```python
from build123d import *

# Parameters (mm, degrees)
F1_DEPTH  = 37
F2_R      = 2
F3_DEPTH  = 25.4
F4_R      = 5
F2_W      = 38.9878123262
F2_H      = 37
F5_DEPTH  = 10
F6_R      = 3
F7_DEPTH  = 10
F9_DEPTH  = 25.4
F11_DEPTH = 25.4


with BuildPart() as f1:
    # F0 (on Front) → F1 (new body)
    with BuildSketch(Plane.XZ):
        with BuildLine():
            Line((-75.544338002, 59.8869249225), (-114.5321503282, 59.8869249225))
            Line((-114.5321503282, 59.8869249225), (-114.5509034395, 46.8869249225))
            Line((-114.5509034395, 46.8869249225), (-110.5809034395, 46.8811980108))
            ThreePointArc((-110.5809034395, 46.8811980108), (-95.048956228, 54.9422402402), (-79.514338002, 46.8863465853))
            Line((-79.514338002, 46.8863465853), (-75.544338002, 46.8863465853))
            Line((-75.544338002, 46.8863465853), (-75.544338002, 59.8869249225))
        make_face()
    extrude(amount=F1_DEPTH)

    # F2 (on face) → F3 (cut)
    with BuildSketch(Plane.XY.offset(59.8869249225)):
        with Locations((-95.0382441651, -18.5)):
            Circle(F2_R)
    extrude(amount=-F3_DEPTH, mode=Mode.SUBTRACT)

    # F4 (on face) + F2 (on face) → F5 (join)
    with BuildSketch(Plane.XY.offset(59.8869249225)):
        with BuildLine():
            Line((-75.544338002, -37), (-61.284338002, -37))
            ThreePointArc((-61.284338002, -37), (-56.4913599263, -18.5), (-61.284338002, 0))
            Line((-61.284338002, 0), (-75.544338002, 0))
            Line((-75.544338002, 0), (-75.544338002, -37))
        make_face()
        with Locations((-69.575338002, -18.5)):
            Circle(F4_R, mode=Mode.SUBTRACT)
        with BuildLine():
            Line((-128.7921503282, -37), (-114.5321503282, -37))
            Line((-114.5321503282, -37), (-114.5321503282, 0))
            Line((-114.5321503282, 0), (-128.7921503282, 0))
            ThreePointArc((-128.7921503282, 0), (-133.6226710865, -18.5), (-128.7921503282, -37))
        make_face()
        with Locations((-120.4896494746, -18.5)):
            Circle(F4_R, mode=Mode.SUBTRACT)
    with BuildSketch(Plane.XY.offset(59.8869249225)):
        with Locations((-95.0382441651, -18.5)):
            Rectangle(F2_W, F2_H)
        with Locations((-95.0382441651, -18.5)):
            Circle(F2_R, mode=Mode.SUBTRACT)
    extrude(amount=F5_DEPTH)

    # F6 (on face) → F7 (join)
    with BuildSketch(Plane.XY.offset(69.8869249225)):
        with BuildLine():
            Line((-75.544338002, 0), (-114.5321503282, 0))
            Line((-114.5321503282, 0), (-114.5321503282, -8.38))
            ThreePointArc((-114.5321503282, -8.38), (-108.9808401176, -18.5), (-114.5321503282, -28.62))
            Line((-114.5321503282, -28.62), (-114.5321503282, -37))
            Line((-114.5321503282, -37), (-75.544338002, -37))
            Line((-75.544338002, -37), (-75.544338002, -28.62))
            ThreePointArc((-75.544338002, -28.62), (-81.0956482126, -18.5), (-75.544338002, -8.38))
            Line((-75.544338002, -8.38), (-75.544338002, 0))
        make_face()
        with Locations((-95.0382441651, -18.5)):
            Circle(F6_R, mode=Mode.SUBTRACT)
    extrude(amount=F7_DEPTH)

    # F8 (on face) → F9 (cut)
    with BuildSketch(Plane(origin=(0, 0, 0), x_dir=(-1, 0, 0), z_dir=(0, 1, 0))):
        with BuildLine():
            ThreePointArc((75.544338002, 69.8869249225), (95.0382441651, 75.2681017907), (114.5321503282, 69.8869249225))
            Line((114.5321503282, 69.8869249225), (114.5321503282, 79.8869249225))
            Line((114.5321503282, 79.8869249225), (75.544338002, 79.8869249225))
            Line((75.544338002, 79.8869249225), (75.544338002, 69.8869249225))
        make_face()
    extrude(amount=-F9_DEPTH, mode=Mode.SUBTRACT)

    # F10 (on face) → F11 (cut)
    with BuildSketch(Plane.XZ.offset(37)):
        with BuildLine():
            ThreePointArc((-114.5321503282, 69.8869249225), (-95.0382441651, 75.2681017907), (-75.544338002, 69.8869249225))
            Line((-75.544338002, 69.8869249225), (-75.544338002, 79.8869249225))
            Line((-75.544338002, 79.8869249225), (-114.5321503282, 79.8869249225))
            Line((-114.5321503282, 79.8869249225), (-114.5321503282, 69.8869249225))
        make_face()
    extrude(amount=-F11_DEPTH, mode=Mode.SUBTRACT)


solid = f1.part
```
Check sheet for the modelled part. Datum: model origin and axes. Units: mm. A direction names the side the tool comes from. Round coordinates to 2 decimals unless told otherwise and drop trailing zeros. Loops run counter-clockwise (first coordinate to the right, second up) from the corner with the lowest first, then second, coordinate; pieces in that order, holes last. Notation, with made-up numbers: (68.25, -6.5) -> (77.25, -6.5) arc R23 cw to (77.25, 7.5) -> close; hole circle Ø8 at (41.5, -18). An arc over 180 degrees is marked (long way). Write item = value, one per line. Start each with the question number.
1) Sectioned sample at C-C, the plane z = 49. Record the cut outline in (x, y), plus the area to 3 significant figures.
2) Sectioned sample at B-B, the plane y = -18.5. State how many separate pieces and enclosed holes the cut face has, plus the area to 3 significant figures.
3) Release check for a two-part mould opening along X. For faces 1 (the flat face through (-75.544, -18, 53)), 2 (the cylindrical face through (-97.419, -20.325, 72.542)), 3 (the flat face through (-127, -18, 69.887)), 4 (the cylindrical face through (-133.62, -18.23, 64.82)) record: released by +X, released by -X, zero draft, split by the parting line, or undercut.
4) Sectioned sample at D-D, the plane x = -123. Record the cut outline in (y, z).
5) Gauge pin test, flat ends, axial feed: pin 1 Ø4.5 at (x, y) = (-95.04, -18.5) entering from -Z; pin 2 Ø1.2 at (x, y) = (-77, -18.5) entering from -Z; pin 3 Ø4 at (y, z) = (-23, 72) entering from +X. Record the tip position at first contact, or that the pin passes through.
6) Thickness scan on probe 1 along Z at (x, y) = (-113, -27); probe 2 along X at (y, z) = (-13, 51.75); probe 3 along X at (y, z) = (-12, 51.5). Record the ranges inside material, lowest first.
7) Sectioned sample at A-A, the plane z = 62. Record the cut outline in (x, y).
8) Set-up check for faces 5 (the flat face through (-95, -16, 69.887)), 6 (the flat face through (-64, -18, 59.887)), 7 (the cylindrical face through (-81.094, -18.669, 70.93)), 8 (the cylindrical face through (-108.982, -18.331, 70.93)): record each of +Z, -Z, +X, -X, +Y, -Y from which the full face is reachable in a straight line by a thin tool's end or side.
Results are:
q1.outline = (-114.55, -37) -> (-108.85, -37) -> (-108.85, 0) -> (-114.55, 0) -> close; (-81.24, -37) -> (-75.54, -37) -> (-75.54, 0) -> (-81.24, 0) -> close
q1.area = 422 mm^2
q2.separate_pieces = 4
q2.enclosed_holes = 0
q2.area = 937 mm^2
q3.face_1 = released by +X
q3.face_2 = undercut
q3.face_3 = zero draft
q3.face_4 = released by -X
q4.outline = (-37, 59.89) -> (-22.82, 59.89) -> (-22.82, 69.89) -> (-37, 69.89) -> close; (-14.18, 59.89) -> (0, 59.89) -> (0, 69.89) -> (-14.18, 69.89) -> close
q5.pin_1 = 54.81
q5.pin_2 = 46.89
q5.pin_3 = -79.19
q6.probe_1 = 46.88 to 69.89
q6.probe_2 = -114.54 to -105.59, -84.5 to -75.54
q6.probe_3 = -114.54 to -105.95, -84.14 to -75.54
q7.outline = (-128.79, -37) -> (-61.28, -37) arc R38.1 ccw to (-61.28, 0) -> (-128.79, 0) arc R37.84 ccw to start; hole circle Ø10 at (-120.49, -18.5); hole circle Ø4 at (-95.04, -18.5); hole circle Ø10 at (-69.58, -18.5)
q8.face_5 = +Z
q8.face_6 = -Z, +X, +Y, -Y
q8.face_7 = +Z, +X
q8.face_8 = +Z, -X
